For this review, use the dimensioned drawing (mm, ordinates from the lowest corner) and the shaded views. A direction names the side the tool comes from. Round coordinates to 2 decimals unless told otherwise and drop trailing zeros. Order: outer loops, then holes, each group sorted by start corner. A loop starts at its lowest first (then second) coordinate and runs counter-clockwise, first axis right, second up. Notation, with made-up numbers: M -31,85 L 12,85 A9 ccw 12,90 Z; hole C 10.5,71.25 d8. An arc over 180 degrees is marked long. Put each result on its own line as item: value.
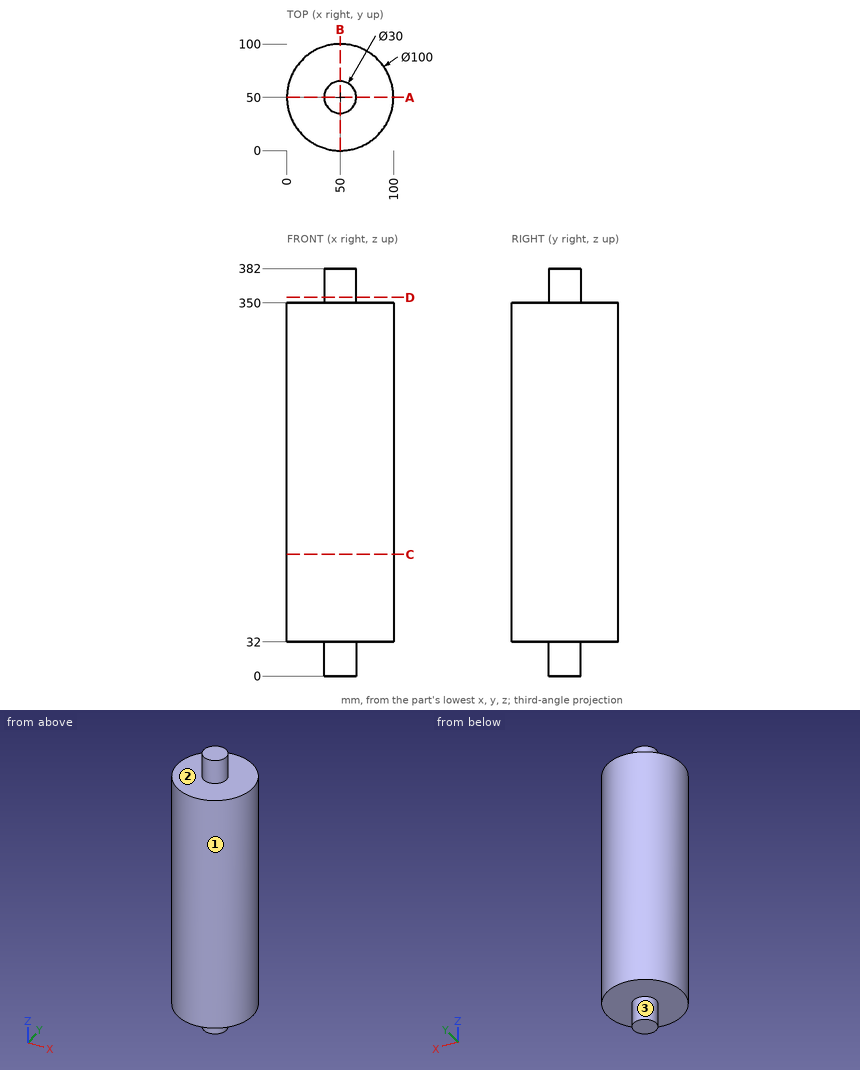
(1) Add section D-D on z = 355. Give the boundary of the cut face in (x, y).
A:
outline: C 50,50 d30
(2) Add section A-A on y = 50. Give the boundary of the cut face in (x, z), then the cut area to 3 significant figures.
A:
outline: M 0,32 L 35,32 L 35,0 L 65,0 L 65,32 L 100,32 L 100,350 L 65,350 L 65,382 L 35,382 L 35,350 L 0,350 Z
area: 33,700 mm2
(3) To check wall thickness, follow L1, parallel to Z at x = 27.5, y = 9; L2, parallel to X at y = 6, z = 222; L3, parallel to Y at x = 44.5, z = 76.5. State the ranges of each line that lie inside material, in increasing order.
A:
L1: z = 32 to 350
L2: x = 26.25 to 73.75
L3: y = 0.3 to 99.7
(4) Insertion check: pin 1 Ø3 at (y, z) = (19.5, 339) entering from +X; pin 2 Ø1 at (x, z) = (73, 312) entering from -Y; pin 3 Ø12 at (y, z) = (23.5, 68) entering from -X; pin 4 Ø8 at (y, z) = (52.5, 78.5) entering from +X. Each pin has a flat end and moves straight along its axis. Give the tip position at first contact, or say it passes through.
A:
pin 1: stops at x = 90.73
pin 2: stops at y = 5.35
pin 3: stops at x = 4.4
pin 4: stops at x = 100
(5) Add section C-C on z = 114. Give the boundary of the cut face in (x, y), then the cut area to 3 significant figures.
A:
outline: C 50,50 d100
area: 7,850 mm2
(6) For the marked faces 1, 2 and 3, list the 3-axis set-ups (+Z, -Z, +X, -X, +Y, -Y) from which the entire face can be reached by the end or side of a thin tool; tool diameter is ignored.
A:
face 1: +Z, -Z
face 2: +Z
face 3: -Z
